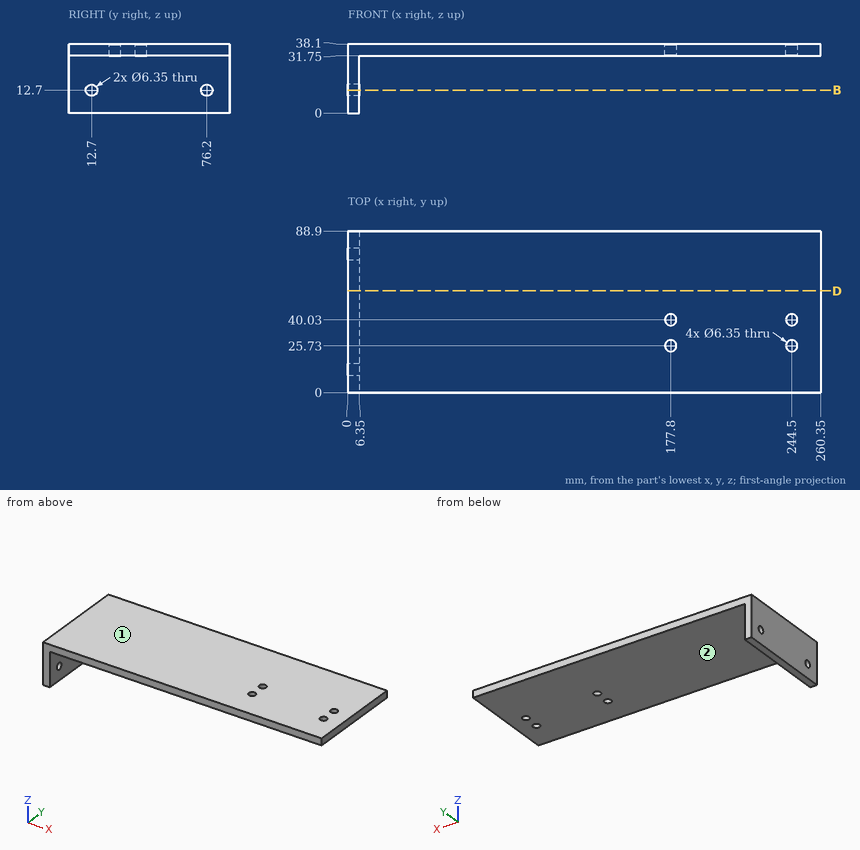
Study the drawing (mm; zero at the part's minimum x, y, z) and answer. A direction names the side the tool comes from. Round coordinates to 2 decimals unless told otherwise and drop trailing zeros. Write each loop counter-clockwise with the first axis right and the second up, starting at its lowest first coordinate (ties: lowest second). Pieces come first, ordered by that corner, then holes. Notation, with made-up numbers: (87.25, -4) -> (103.25, -4) arc R20 cw to (103.25, 17) -> close; hole circle Ø4 at (52, -8.75). An arc over 180 degrees is marked (long way). Write each question's results on one line, items separated by ' | '.
Item 1: Find the intervals of material crossed by line 1 along Y through (x, z) = (177.8, 33.25) (1 decimal); line 2 along Y through (x, z) = (4, 12); line 3 along Z through (x, y) = (3.75, 76.2) (1 decimal), in increasing order. Write a range as [from, to].
Result set:
line 1: [0, 22.6], [28.9, 36.9], [43.2, 88.9] | line 2: [0, 9.6], [15.8, 73.1], [79.3, 88.9] | line 3: [0, 9.5], [15.9, 38.1]
Item 2: Which of the six approach directions +Z, -Z, +X, -X, +Y, -Y give full straight-line access (tool end or side, diameter ignored) to the marked faces 1 and 2?
Result set:
face 1: +Z, +X, -X, +Y, -Y | face 2: -Z, +X, +Y, -Y
Item 3: Flat-ended cylindrical pins translate along their axes: P1, Ø1, axis at y = 41, z = 4, coming from the +X side; P2, Ø4, axis at x = 177.8, y = 25.73, coming from the -Z side; P3, Ø10, axis at x = 244.5, y = 25.73, coming from the -Z side. Find the tip coordinate at first contact, or state that the pin passes through.
Result set:
P1: x = 6.35 | P2: through | P3: z = 31.75
Item 4: A cutting plane is placed at B-B, the plane z = 12.7. Count the separate pieces of the cut face and the enclosed holes in it, plus the area to 3 significant figures.
Result set:
separate pieces: 3 | enclosed holes: 0 | area: 484 mm^2
Item 5: A cutting plane is placed at D-D, the plane y = 56. Determine the outline of the cut face in (x, z).
Result set:
outline: (0, 0) -> (6.35, 0) -> (6.35, 31.75) -> (260.35, 31.75) -> (260.35, 38.1) -> (0, 38.1) -> close
